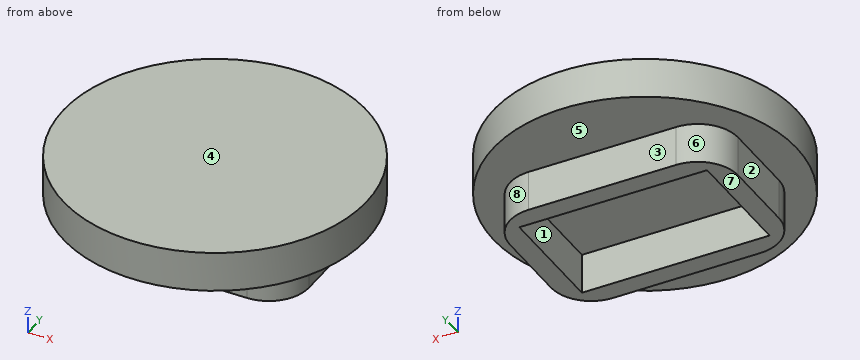
from build123d import *

# Parameters (mm, degrees)
SKETCH1_R           = 37.5
BOSS_EXTRUDE1_DEPTH = 10
BOSS_EXTRUDE2_DEPTH = 10


with BuildPart() as part:
    # Sketch1 → Boss-Extrude1 (new body)
    with BuildSketch(Plane.XY):
        with Locations((11.945516858, 0)):
            Circle(SKETCH1_R)
    extrude(amount=BOSS_EXTRUDE1_DEPTH)

    # Sketch2 → Boss-Extrude2 (add)
    with BuildSketch(Plane(origin=(0, 0, 0), x_dir=(-1, 0, 0), z_dir=(0, 0, -1))):
        with BuildLine():
            Line((-30.25, 19.484324941), (6.25, 19.484324941))
            ThreePointArc((6.25, 19.484324941), (13.321067812, 16.555392753), (16.25, 9.484324941))
            Line((16.25, 9.484324941), (16.25, -9.205373472))
            ThreePointArc((16.25, -9.205373472), (13.324868437, -16.272638614), (6.260752682, -19.205367691))
            Line((6.260752682, -19.205367691), (-30.239247318, -19.244615001))
            ThreePointArc((-30.239247318, -19.244615001), (-37.317265142, -16.319489219), (-40.25, -9.244620782))
            Line((-40.25, -9.244620782), (-40.25, 9.484324941))
            ThreePointArc((-40.25, 9.484324941), (-37.321067812, 16.555392753), (-30.25, 19.484324941))
        make_face()
        Polygon((-35.25, -14.250000016), (11.25, -14.200000018), (11.25, 14.484324941), (-35.25, 14.484324941), align=None, mode=Mode.SUBTRACT)
    extrude(amount=BOSS_EXTRUDE2_DEPTH)


solid = part.part
Geometry: final body of the model. Coordinates: model frame, mm. Face numbers are marked on the shaded views. A direction names the side the tool comes from. Round coordinates to 2 decimals unless told otherwise and drop trailing zeros. Loops run counter-clockwise (first coordinate to the right, second up) from the corner with the lowest first, then second, coordinate; pieces in that order, holes last. Notation, with made-up numbers: (65, 32) - (99, 32) arc R17 cw to (99, 45) - close; hole circle Ø6 at (9, 39). An arc over 180 degrees is marked (long way). Write each question's results on one line, items separated by ' | '. Start each with the question number.
1) Cut plane B-B on y = 0. Return loops of the section in (x, z).
2) Cut plane A-A on z = -4.75. Return loops of the section in (x, y).
3) Cut plane D-D on z = 8.5. Return loops of the section in (x, y).
4) Line query: probe 1 along Y at (x, z) = (4.5, -1.75); probe 2 along Z at (x, y) = (7, -9); probe 3 along Y at (x, z) = (-9.5, -4.75). Output: solid intervals per line, ascending. Write a range as [from, to].
5) Mould query, pull axis Y, two halves, no side actions, for the marked faces 1, 2 and 3. Classes: released by +Y, released by -Y, zero draft, split by the parting line, or undercut.
6) First-contact query: P1, Ø8, axis at y = 6, z = -5, coming from the +X side; P2, Ø1, axis at x = 11, z = -3.5, coming from the +Y side; P3, Ø10, axis at y = -12.5, z = -8, coming from the -X side. Flat tips, straight axial feed; report the tip coordinate or a pass-through.
7) Cut plane C-C on x = 27.5. Return loops of the section in (y, z).
8) Access query for the marked faces 4, 5, 6, 7 and 8. Directions: +Z, -Z, +X, -X, +Y, -Y. A direction counts if a zero-diameter tool reaches every point of the face in a straight line with its end or side. Return the directions, or none.
Verdict:
1) outline: (-25.55, 0) - (-16.25, 0) - (-16.25, -10) - (-11.25, -10) - (-11.25, 0) - (35.25, 0) - (35.25, -10) - (40.25, -10) - (40.25, 0) - (49.45, 0) - (49.45, 10) - (-25.55, 10) - close
2) outline: (-16.25, -9.21) arc R10 ccw to (-6.26, -19.21) - (30.24, -19.24) arc R10 ccw to (40.25, -9.24) - (40.25, 9.48) arc R10 ccw to (30.25, 19.48) - (-6.25, 19.48) arc R10 ccw to (-16.25, 9.48) - close; hole (-11.25, -14.2) - (35.25, -14.25) - (35.25, 14.48) - (-11.25, 14.48) - close
3) outline: circle Ø75 at (11.95, 0)
4) probe 1: y = [-19.22, -14.22], [14.48, 19.48] | probe 2: z = [0, 10] | probe 3: y = [-18.66, -14.2], [14.48, 18.94]
5) face 1: undercut | face 2: zero draft | face 3: released by +Y
6) P1: stops at x = 40.25 | P2: stops at y = 19.48 | P3: stops at x = -16.25
7) outline: (-34.12, 0) - (-19.24, 0) - (-19.24, -10) - (-14.24, -10) - (-14.24, 0) - (14.48, 0) - (14.48, -10) - (19.48, -10) - (19.48, 0) - (34.12, 0) - (34.12, 10) - (-34.12, 10) - close
8) face 4: +Z, +X, -X, +Y, -Y | face 5: -Z | face 6: -Z, -X, +Y | face 7: -Z, +X, -X, +Y, -Y | face 8: -Z, +X, +Y
